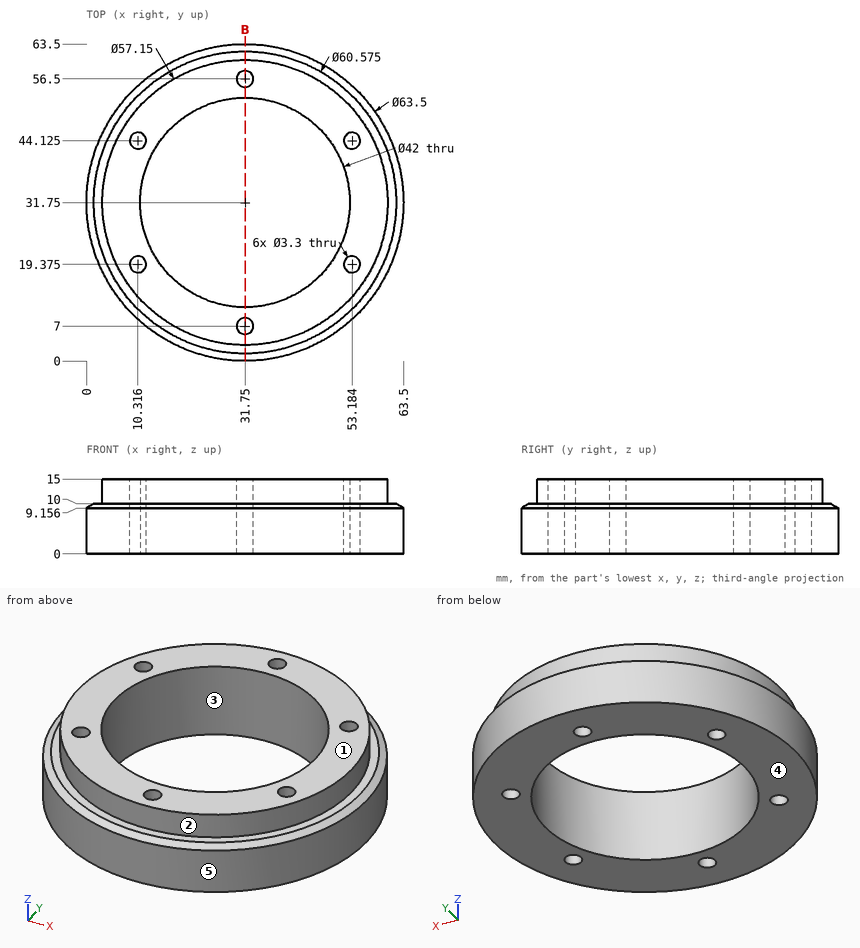
Source: three-view drawing plus pictorial views. Frame: mm from the lowest corner of the part. A direction names the side the tool comes from. Give positions to 0.01 mm unless a question says otherwise; leave off trailing zeros. Write item = value, one per line. Start each with the question number.
1. Ray query, L1, parallel to X at y = 31.5, z = 13.25; L2, parallel to X at y = 19, z = 8 (1 decimal); L3, parallel to X at y = 44, z = 8.25. Return the intervals inside material, ascending.
2. Access query for the marked faces 1 and 2. Directions: +Z, -Z, +X, -X, +Y, -Y. A direction counts if a zero-diameter tool reaches every point of the face in a straight line with its end or side. Return the directions, or none.
3. First-contact query: pin 1 Ø8 at (x, z) = (54, 3.5) entering from +Y; pin 2 Ø1.5 at (x, z) = (29, 9) entering from +Y; pin 3 Ø3 at (x, z) = (20, 4) entering from -Y. Flat tips, straight axial feed; report the tip coordinate or a pass-through.
4. Section query B-B, the plane x = 31.75. Count the separate pieces of the cut face and the enclosed holes in it.
5. Mould query, pull axis Y, two halves, no side actions, for the marked faces 3, 4 and 5. Classes: released by +Y, released by -Y, zero draft, split by the parting line, or undercut.
Check sheet entries:
q1.L1 = 3.18 to 10.75, 52.75 to 60.32
q1.L2 = 2.7 to 8.7, 11.9 to 15.1, 48.4 to 51.6, 54.8 to 60.8
q1.L3 = 2.46 to 8.67, 11.96 to 14.69, 48.81 to 51.54, 54.83 to 61.04
q2.face_1 = +Z, +X, -X, +Y, -Y
q2.face_2 = +Z
q3.pin_1 = 57.73
q3.pin_2 = 63.44
q3.pin_3 = 1.7
q4.separate_pieces = 4
q4.enclosed_holes = 0
q5.face_3 = undercut
q5.face_4 = zero draft
q5.face_5 = split by the parting line
